Source: CAD feature listing. Evaluate the final solid. Frame: model axes, mm. A direction names the side the tool comes from. Give positions to 0.01 mm unless a question says otherwise; leave off trailing zeros. Order: outer loops, then holes, each group sorted by start corner. A loop starts at its lowest first (then second) coordinate and runs counter-clockwise, first axis right, second up.
```python
from build123d import *

# Parameters (mm, degrees)
F0_W     = 300
F0_H     = 110
F1_DEPTH = 25
F2_R     = 5
F3_DEPTH = 15
F4_R     = 15
F5_R     = 5


with BuildPart() as f1:
    # F0 (on Top) → F1 (new body)
    with BuildSketch(Plane.XY):
        Rectangle(F0_W, F0_H)
    extrude(amount=F1_DEPTH)

    # F2 (on face) → F3 (cut)
    with BuildSketch(Plane(origin=(0, 0, 0), x_dir=(1, 0, 0), z_dir=(0, 0, -1))):
        with Locations((-112.5, 35)):
            Circle(F2_R)
        with Locations((112.5, 35)):
            Circle(F2_R)
        with Locations((112.5, -35)):
            Circle(F2_R)
        with Locations((-112.5, -35)):
            Circle(F2_R)
    extrude(amount=-F3_DEPTH, mode=Mode.SUBTRACT)

    # F4
    f4_edges = [f1.edges().sort_by_distance(p)[0] for p in [
        (-150, 55, 12.5),
        (-150, -55, 12.5),
        (150, -55, 12.5),
        (150, 55, 12.5),
    ]]
    fillet(f4_edges, radius=F4_R)

    # F5
    f5_edges = [f1.edges().sort_by_distance(p)[0] for p in [
        (-150, 0, 25),
        (-150, 0, 0),
    ]]
    fillet(f5_edges, radius=F5_R)


solid = f1.part
```
1) Section query A-A, the plane z = 11.75. Return the cut outline in (x, y), and give its area (3 significant figures).
Report:
outline: (-150, -40) arc R15 ccw to (-135, -55) - (135, -55) arc R15 ccw to (150, -40) - (150, 40) arc R15 ccw to (135, 55) - (-135, 55) arc R15 ccw to (-150, 40) - close; hole circle Ø10 at (-112.5, -35); hole circle Ø10 at (-112.5, 35); hole circle Ø10 at (112.5, -35); hole circle Ø10 at (112.5, 35)
area: 32,500 mm2
2) Section query B-B, the plane y = -35. Return the cut outline in (x, z).
Report:
outline: (-150, 5) arc R5 ccw to (-145, 0) - (-117.5, 0) - (-117.5, 15) - (-107.5, 15) - (-107.5, 0) - (107.5, 0) - (107.5, 15) - (117.5, 15) - (117.5, 0) - (145, 0) arc R5 ccw to (150, 5) - (150, 20) arc R5 ccw to (145, 25) - (-145, 25) arc R5 ccw to (-150, 20) - close
3) Pin query (flat end, axial travel): pin 1 (3 mm diameter, centred on x = 111.5, y = -37, fed in from -Z); pin 2 (2 mm diameter, centred on x = 107, z = 3.5, fed in from -Y). Return the tip coordinate at first contact, or that it passes through.
Report:
pin 1: stops at z = 15
pin 2: stops at y = -54.97
4) Draft query along X for faces 3 (the cylindrical face through (117.119, 36.915, 7.395)), 4 (the flat face through (112, -35, 15)), 5 (the cylindrical face through (-2, -54, 23)), 6 (the cylindrical face through (149, -1, 23)). Return one class per face: +X half, -X half, draft (parallel to the pull), parting line (faces both ways), or undercut.
Report:
face 3: undercut
face 4: undercut
face 5: draft
face 6: +X half
5) Section query C-C, the plane x = 112.5. Return the cut outline in (y, z).
Report:
outline: (-55, 5) arc R5 ccw to (-50, 0) - (-40, 0) - (-40, 15) - (-30, 15) - (-30, 0) - (30, 0) - (30, 15) - (40, 15) - (40, 0) - (50, 0) arc R5 ccw to (55, 5) - (55, 20) arc R5 ccw to (50, 25) - (-50, 25) arc R5 ccw to (-55, 20) - close
6) Material intervals for L1, parallel to X at y = -35, z = 6; L2, parallel to Y at x = -112.5, z = 6; L3, parallel to Y at x = 112.5, z = 4, sorted ascending.
Report:
L1: x = -150 to -117.5, -107.5 to 107.5, 117.5 to 150
L2: y = -55 to -40, -30 to 30, 40 to 55
L3: y = -54.9 to -40, -30 to 30, 40 to 54.9
7) Reachability of faces 1 (the cylindrical face through (-145.72, -50.49, 12.6)), 2 (the flat face through (-113, -35, 15)) from +Z, -Z, +X, -X, +Y, -Y: full face, straight path, thin tool, end or side. Return the list, or none.
Report:
face 1: +Z, -Z, -X, -Y
face 2: -Z
